CAD build for the part. Positions are in the model's coordinates, mm. A direction names the side the tool comes from. Coordinates: 2 decimals unless noted, no trailing zeros. Loops run counter-clockwise (first coordinate to the right, second up) from the corner with the lowest first, then second, coordinate; pieces in that order, holes last.
1) Saw through at A-A, the plane x = 0. Write the cut outline in (y, z).
2) Pin check, flat tips, straight feed: pin 1 Ø4.5 at (x, y) = (-5, 13) entering from -Z; pin 2 Ø2.5 at (x, z) = (1, -5.5) entering from +Y; pin 3 Ø1 at (y, z) = (6.5, 0.5) entering from -X. Stop position of each tip, or through.
3) Saw through at D-D, the plane x = -9.25. Write the cut outline in (y, z), and give its area (3 significant figures).
4) Wall check: line 1 along Z through (x, y) = (-1.5, 15.75); line 2 along Y through (x, z) = (0.25, -5); line 3 along X through (y, z) = (1.75, -4.25). Give the ranges that are in metal, low to high.
5) Saw through at C-C, the plane y = 8. Write the cut outline in (x, z), and give its area (3 significant figures).
6) Two-plate mould, pull along X, no slides. Class faces 1 (the cylindrical face through (12.4, 21.43, -0.04)), 2 (the flat face through (0, 16, -2.5)), 3 (the flat face through (-1.8, 2, 0)): +X half, -X half, draft (parallel to the pull), parting line (faces both ways), or undercut.
7) Saw through at B-B, the plane z = 0. Write the cut outline in (x, y), and give its area (3 significant figures).
8) Which spindle directions (+Z, -Z, +X, -X, +Y, -Y) get a long thin tool onto all of the face, cutting with end or side? Do faces 4 (the flat face through (0, 3.2, 0)), 5 (the cylindrical face through (2.834, 3.746, 6.836)), 6 (the flat face through (0, 7, -6)), 7 (the flat face through (0, 7, 6)), 8 (the cylindrical face through (-12.43, 21.4, -0.04)). Say none if no direction does.
```python
from build123d import *

# Parameters (mm, degrees)
SKETCH1_R           = 7.4
BOSS_EXTRUDE1_DEPTH = 7
SKETCH2_W           = 3.6
SKETCH2_H           = 16.327847923
CUT_EXTRUDE1_DEPTH  = 3.2
FILLET1_R           = 0.5
SKETCH3_W           = 26
SKETCH3_H           = 5
BOSS_EXTRUDE2_DEPTH = 15
CUT_EXTRUDE2_DEPTH  = 28.404561664
FILLET2_R           = 2
FILLET3_R           = 2


with BuildPart() as part:
    # Sketch1 → Boss-Extrude1 (new body)
    with BuildSketch(Plane(origin=(0, 0, 0), x_dir=(1, 0, 0), z_dir=(0, 1, 0))):
        with Locations(Location((0, 0, 0), (0, 0, 270))):
            Circle(SKETCH1_R)
    extrude(amount=BOSS_EXTRUDE1_DEPTH)

    # Sketch2 → Cut-Extrude1 (cut)
    with BuildSketch(Plane.XZ):
        with Locations((0, -0.126477582)):
            Rectangle(SKETCH2_W, SKETCH2_H)
    extrude(amount=-CUT_EXTRUDE1_DEPTH, mode=Mode.SUBTRACT)

    # Fillet1
    fillet1_edges = [part.edges().sort_by_distance(p)[0] for p in [
        (7.4, 0, 0),
        (-7.4, 0, 0),
        (1.8, 0, 0),
        (-1.8, 0, 0),
    ]]
    fillet(fillet1_edges, radius=FILLET1_R)

    # Sketch3 → Boss-Extrude2 (add)
    with BuildSketch(Plane(origin=(0, 7, 0), x_dir=(1, 0, 0), z_dir=(0, 1, 0))):
        Rectangle(SKETCH3_W, SKETCH3_H)
    extrude(amount=BOSS_EXTRUDE2_DEPTH)

    # Sketch4 → Cut-Extrude2 (cut, through all)
    with BuildSketch(Plane.XY.offset(2.5)):
        Polygon((-6.96491206, 7), (-13, 17), (-13, 7), align=None)
        Polygon((6.96491206, 7), (13, 17), (13, 7), align=None)
    extrude(amount=-CUT_EXTRUDE2_DEPTH, mode=Mode.SUBTRACT)

    # Fillet2
    fillet2_edges = [part.edges().sort_by_distance(p)[0] for p in [
        (-13, 22, 0),
        (13, 22, 0),
    ]]
    fillet(fillet2_edges, radius=FILLET2_R)

    # Fillet3
    # the kernel refuses this fillet: 2 mm, written as the material it adds along each edge
    with BuildSketch(Plane(origin=(11.96491206, 7, 2.5), x_dir=(0, 1, 0), z_dir=(-1, 0, 0))) as fillet3_piece_1_section:
        with BuildLine():
            CenterArc((FILLET3_R, -FILLET3_R), FILLET3_R, 90, 90)
            Line((0, -FILLET3_R), (0, 0))
            Line((0, 0), (FILLET3_R, 0))
        make_face()
    fillet3_piece_1 = extrude(amount=23.929824119, mode=Mode.PRIVATE)
    fillet3_piece_1 = fillet3_piece_1 & Plane(origin=(0, 7.46029714, 0), x_dir=(0, 0, 1), z_dir=(0, -1, 0)) * Cylinder(7.4, 56, mode=Mode.PRIVATE)
    add(fillet3_piece_1)
    with BuildSketch(Plane(origin=(-11.96491206, 7, -2.5), x_dir=(0, 1, 0), z_dir=(1, 0, 0))) as fillet3_piece_2_section:
        with BuildLine():
            CenterArc((FILLET3_R, -FILLET3_R), FILLET3_R, 90, 90)
            Line((0, -FILLET3_R), (0, 0))
            Line((0, 0), (FILLET3_R, 0))
        make_face()
    fillet3_piece_2 = extrude(amount=23.929824119, mode=Mode.PRIVATE)
    fillet3_piece_2 = fillet3_piece_2 & Plane(origin=(0, 7.460297172, 0), x_dir=(0, 0, 1), z_dir=(0, -1, 0)) * Cylinder(7.4, 56, mode=Mode.PRIVATE)
    add(fillet3_piece_2)


solid = part.part
```
Data:
1. outline: (3.2, -7.4) - (7, -7.4) - (7, -4.5) arc R2 cw to (9, -2.5) - (22, -2.5) - (22, 2.5) - (9, 2.5) arc R2 cw to (7, 4.5) - (7, 7.4) - (3.2, 7.4) - close
2. pin 1: stops at z = -2.5
2. pin 2: stops at y = 7.02
2. pin 3: stops at x = -7.4
3. outline: (10.79, -2.5) - (22, -2.5) - (22, 2.5) - (10.79, 2.5) - close
3. area: 56.1 mm2
4. line 1: z = -2.5 to 2.5
4. line 2: y = 3.2 to 7
4. line 3: x = -6.06 to -1.8, 1.8 to 6.06
5. outline: (-7.57, -2.5) - (-6.96, -2.5) arc R7.4 ccw to (-6.86, -2.77) - (6.86, -2.77) arc R7.4 ccw to (6.96, -2.5) - (7.57, -2.5) - (7.57, 2.5) - (6.96, 2.5) arc R7.4 ccw to (6.86, 2.77) - (-6.86, 2.77) arc R7.4 ccw to (-6.96, 2.5) - (-7.57, 2.5) - close
5. area: 83.1 mm2
6. face 1: +X half
6. face 2: draft
6. face 3: undercut
7. outline: (-13, 17) - (-6.96, 7) - (-7.4, 7) - (-7.4, 0.5) arc R0.5 ccw to (-6.9, 0) - (-2.3, 0) arc R0.5 ccw to (-1.8, 0.5) - (-1.8, 3.2) - (1.8, 3.2) - (1.8, 0.5) arc R0.5 ccw to (2.3, 0) - (6.9, 0) arc R0.5 ccw to (7.4, 0.5) - (7.4, 7) - (6.96, 7) - (13, 17) - (13, 20) arc R2 ccw to (11, 22) - (-11, 22) arc R2 ccw to (-13, 20) - close
7. area: 420 mm2
8. face 4: +Z, -Z, -Y
8. face 5: -Y
8. face 6: -Z, +X, -X, +Y
8. face 7: +Z, +X, -X, +Y
8. face 8: +Z, -Z, -X, +Y
